For this review, take the finished solid that the model builds, in its own axes (mm). Give positions to 0.01 mm unless a question says otherwise; leave off trailing zeros. Order: outer loops, then holes, each group sorted by start corner. A loop starts at its lowest first (then second) coordinate and runs counter-clockwise, first axis right, second up.
from build123d import *

# Parameters (mm, degrees)
SKETCH1_R               = 114.3
BOSS_EXTRUDE2_DEPTH     = 4.064
CUT_EXTRUDE1_DEPTH      = 70.612
CUT_EXTRUDE1_DEPTH_BACK = 101.6
SKETCH3_R               = 12.7
SKETCH4_R               = 2.9972
CUT_EXTRUDE3_DEPTH      = 70.612


with BuildPart() as part:
    # Sketch1 → Boss-Extrude2 (new body)
    with BuildSketch(Plane.XY):
        Circle(SKETCH1_R)
    extrude(amount=BOSS_EXTRUDE2_DEPTH)

    # Sketch3 → Cut-Extrude1 (cut, two sides: drawn at the far end of the back side and taken through both)
    with BuildSketch(Plane.XY.offset(4.064).offset(-CUT_EXTRUDE1_DEPTH_BACK)):
        Circle(SKETCH3_R)
    extrude(amount=CUT_EXTRUDE1_DEPTH + CUT_EXTRUDE1_DEPTH_BACK, mode=Mode.SUBTRACT)

    # Sketch4 → Cut-Extrude3 (cut)
    with BuildSketch(Plane.XY.offset(4.064)):
        with Locations((0, -24.638)):
            Circle(SKETCH4_R)
        with Locations((-21.337133898, -12.319)):
            Circle(SKETCH4_R)
        with Locations((-21.337133898, 12.319)):
            Circle(SKETCH4_R)
        with Locations((0, 24.638)):
            Circle(SKETCH4_R)
        with Locations((21.337133898, 12.319)):
            Circle(SKETCH4_R)
        with Locations((21.337133898, -12.319)):
            Circle(SKETCH4_R)
    extrude(amount=-CUT_EXTRUDE3_DEPTH, mode=Mode.SUBTRACT)


solid = part.part
1) Draft analysis for pull direction X (two halves, no side actions). For faces 1 (the face through (24, 2, 4.064)), 2 (the face through (-114.19, 5.03, 2)), 3 (the face through (24.106, -13.467, 2.06)), 4 (the face through (1.61, -22.11, 2.06)), state which applies: +X half, -X half, draft (parallel to the pull), parting line (faces both ways), or undercut.
Answer sheet:
face 1: draft
face 2: parting line
face 3: undercut
face 4: undercut
2) We need section A-A on x = 0. Give the boundary of the cut face in (y, z), then the cut area to 3 significant figures.
Answer sheet:
outline: (-114.3, 0) - (-27.64, 0) - (-27.64, 4.06) - (-114.3, 4.06) - close; (-21.64, 0) - (-12.7, 0) - (-12.7, 4.06) - (-21.64, 4.06) - close; (12.7, 0) - (21.64, 0) - (21.64, 4.06) - (12.7, 4.06) - close; (27.64, 0) - (114.3, 0) - (114.3, 4.06) - (27.64, 4.06) - close
area: 777 mm2
3) Clearance check with flat-ended pins moving along their axes: pin 1 (1.5 mm diameter, centred on x = 41, z = 2.5, fed in from +Y); pin 2 (1.5 mm diameter, centred on y = -40, z = 2.5, fed in from +X); pin 3 (1.5 mm diameter, centred on y = 44.5, z = 1.5, fed in from -X). State where each tip first meets the part, or that it passes through.
Answer sheet:
pin 1: stops at y = 106.98
pin 2: stops at x = 107.35
pin 3: stops at x = -105.6
4) We need section B-B on z = 3.4. Give the boundary of the cut face in (x, y).
Answer sheet:
outline: circle Ø228.6 at (0, 0); hole circle Ø5.99 at (-21.34, -12.32); hole circle Ø5.99 at (-21.34, 12.32); hole circle Ø25.4 at (0, 0); hole circle Ø5.99 at (0, -24.64); hole circle Ø5.99 at (0, 24.64); hole circle Ø5.99 at (21.34, -12.32); hole circle Ø5.99 at (21.34, 12.32)
5) We need section C-C on y = -61.5. Give the boundary of the cut face in (x, z), then the cut area to 3 significant figures.
Answer sheet:
outline: (-96.34, 0) - (96.34, 0) - (96.34, 4.06) - (-96.34, 4.06) - close
area: 783 mm2
6) We need section D-D on x = 54. Give the boundary of the cut face in (y, z), then the cut area to 3 significant figures.
Answer sheet:
outline: (-100.74, 0) - (100.74, 0) - (100.74, 4.06) - (-100.74, 4.06) - close
area: 819 mm2
7) To check wall thickness, follow line 1 (Y direction, x = 0, z = 2.65); line 2 (X direction, y = -1, z = 1.05); line 3 (Y direction, x = -24, z = 3.8). State the ranges of each line that lie inside material, in increasing order.
Answer sheet:
line 1: y = -114.3 to -27.64, -21.64 to -12.7, 12.7 to 21.64, 27.64 to 114.3
line 2: x = -114.3 to -12.66, 12.66 to 114.3
line 3: y = -111.75 to -13.69, -10.94 to 10.94, 13.69 to 111.75
